Geometry check sheet. Reference: the model listing, model coordinates, mm. Coordinates: 2 decimals unless noted, no trailing zeros. Order: outer loops, then holes, each group sorted by start corner. A loop starts at its lowest first (then second) coordinate and runs counter-clockwise, first axis right, second up.
```python
from build123d import *

# Parameters (mm, degrees)
EXTRUDE_1_DEPTH = 2


with BuildPart() as part:
    # Эскиз1 → Бобышка-Вытянуть1 (new body)
    with BuildSketch(Plane.XY):
        with BuildLine():
            Line((43.587168574, -16.504809472), (44.80864708, -17.210030416))
            ThreePointArc((44.80864708, -17.210030416), (47.195418527, -8.751712409), (48, 0))
            ThreePointArc((48, 0), (36.496575182, 31.176914536), (7.5, 47.410441888))
            Line((7.5, 47.410441888), (7.5, 46))
            Line((7.5, 46), (-7.5, 46))
            Line((-7.5, 46), (-7.5, 47.410441888))
            ThreePointArc((-7.5, 47.410441888), (-41.569219382, 24), (-44.80864708, -17.210030416))
            Line((-44.80864708, -17.210030416), (-43.587168574, -16.504809472))
            Line((-43.587168574, -16.504809472), (-36.087168574, -29.495190528))
            Line((-36.087168574, -29.495190528), (-37.30864708, -30.200411472))
            ThreePointArc((-37.30864708, -30.200411472), (0, -48), (37.30864708, -30.200411472))
            Line((37.30864708, -30.200411472), (36.087168574, -29.495190528))
            Line((36.087168574, -29.495190528), (43.587168574, -16.504809472))
        make_face()
    extrude(amount=EXTRUDE_1_DEPTH)


solid = part.part
```
Item 1: Sectioned sample at C-C (x = -2). Record the cut outline in (y, z).
Item 2: Sectioned sample at B-B (y = -34). Record the cut outline in (x, z), and give its area (3 significant figures).
Item 3: Thickness scan on line 1 along X through (y, z) = (1, 0.6); line 2 along Y through (x, z) = (0, 1.4); line 3 along Y through (x, z) = (36.5, 1.6). Record the ranges inside material, lowest first.
Item 4: Sectioned sample at A-A (z = 0.95). Record the cut outline in (x, y).
Item 5: Depth check by flat-ended pin: P1, Ø0.6, axis at x = 3.5, z = 1, coming from the +Y side. Enter the tip coordinate at first touch or a pass-through.
Geometry check:
1. outline: (-47.96, 0) - (46, 0) - (46, 2) - (-47.96, 2) - close
2. outline: (-33.88, 0) - (33.88, 0) - (33.88, 2) - (-33.88, 2) - close
2. area: 136 mm2
3. line 1: x = -47.99 to 47.99
3. line 2: y = -48 to 46
3. line 3: y = -31.17 to -29.73, -28.78 to 31.17
4. outline: (-44.81, -17.21) - (-43.59, -16.5) - (-36.09, -29.5) - (-37.31, -30.2) arc R48 ccw to (37.31, -30.2) - (36.09, -29.5) - (43.59, -16.5) - (44.81, -17.21) arc R48 ccw to (7.5, 47.41) - (7.5, 46) - (-7.5, 46) - (-7.5, 47.41) arc R48 ccw to start
5. P1: stops at y = 46
